Work out the finished part from the listing and answer in its coordinate system (mm). A direction names the side the tool comes from. Round coordinates to 2 decimals unless told otherwise and drop trailing zeros. Write each loop counter-clockwise with the first axis right and the second up, starting at its lowest first coordinate (ties: lowest second). Pieces come first, ordered by that corner, then holes.
1. Find section B-B (x = 37.5). Write down the section's boundary in (y, z).
2. Find section A-A (y = -10). Write down the section's boundary in (x, z), and give its area (3 significant figures).
3. Straight lines are drawn through the part: probe 1 along X at (y, z) = (12, 3.15); probe 2 along Y at (x, z) = (20, 1.75); probe 3 along X at (y, z) = (18, 2.25). For each, find the intervals that lie inside material, in ascending order.
4. A tool of negligible diameter and unlimited length cuts with its end or side. For faces 1 (the face through (-35, 10, 3)), 2 (the face through (-90, -1, 2)), 3 (the face through (-69.5, 17, 3)), from which of +Z, -Z, +X, -X, +Y, -Y can it reach the whole face along a straight path? Write none if from no direction.
5. Find section C-C (x = -20). Write down the section's boundary in (y, z).
6. Flat-ended cylindrical pins translate along their axes: pin 1 Ø1.5 at (x, z) = (-80.5, 1.5) entering from +Y; pin 2 Ø2.5 at (y, z) = (16.5, 2.5) entering from +X. Find the tip coordinate at first contact, or state that the pin passes through.
7. Determine the mould class of faces 4 (the face through (69.5, 17, 3)), 5 (the face through (1.183, -8.145, 2.535)), 6 (the face through (80, 14, 3)), 7 (the face through (72.1, 5.66, 2.54)) for opening direction X: pulls with the +X half, pulls with the -X half, needs draft (parallel to the pull), parting line crosses it, or undercut.
```python
from build123d import *

# Parameters (mm, degrees)
SZKIC1_W                    = 180
SZKIC1_H                    = 40
DODANIE_WYCI_GNI_CIE1_DEPTH = 5
ZAOKR_GLENIE1_R             = 5
SZKIC2_R                    = 2.2
WYTNIJ_WYCI_GNI_CIE1_DEPTH  = 5
SZKIC3_W                    = 20.5
SZKIC3_H                    = 6
WYTNIJ_WYCI_GNI_CIE2_DEPTH  = 10
SZKIC4_R                    = 2.2
WYTNIJ_WYCI_GNI_CIE3_DEPTH  = 10
SZKIC5_W                    = 12
SZKIC5_H                    = 6
WYTNIJ_WYCI_GNI_CIE4_DEPTH  = 93.330926563
ZAOKR_GLENIE2_R             = 2


with BuildPart() as part:
    # Szkic1 → Dodanie-wyciągnięcie1 (new body)
    with BuildSketch(Plane.XY):
        Rectangle(SZKIC1_W, SZKIC1_H)
    extrude(amount=DODANIE_WYCI_GNI_CIE1_DEPTH)

    # Zaokrąglenie1
    zaokr_glenie1_edges = [part.edges().sort_by_distance(p)[0] for p in [
        (90, -20, 2.5),
        (-90, -20, 2.5),
        (-90, 20, 2.5),
        (90, 20, 2.5),
    ]]
    fillet(zaokr_glenie1_edges, radius=ZAOKR_GLENIE1_R)

    # Szkic2 → Wytnij-wyciągnięcie1 (cut)
    with BuildSketch(Plane.XY.offset(5)):
        with Locations((-70, 5)):
            Circle(SZKIC2_R)
        with Locations((-20, 10)):
            Circle(SZKIC2_R)
        with Locations((20, 10)):
            Circle(SZKIC2_R)
        with Locations((70, 5)):
            Circle(SZKIC2_R)
    extrude(amount=-WYTNIJ_WYCI_GNI_CIE1_DEPTH, mode=Mode.SUBTRACT)

    # Szkic3 → Wytnij-wyciągnięcie2 (cut)
    with BuildSketch(Plane.XY.offset(5)):
        with Locations((-79.75, 17)):
            Rectangle(SZKIC3_W, SZKIC3_H)
        with Locations((79.75, 17)):
            Rectangle(SZKIC3_W, SZKIC3_H)
    extrude(amount=-WYTNIJ_WYCI_GNI_CIE2_DEPTH, mode=Mode.SUBTRACT)

    # Szkic4 → Wytnij-wyciągnięcie3 (cut)
    with BuildSketch(Plane.XY.offset(5)):
        with Locations((0, -10)):
            Circle(SZKIC4_R)
    extrude(amount=-WYTNIJ_WYCI_GNI_CIE3_DEPTH, mode=Mode.SUBTRACT)

    # Szkic5 → Wytnij-wyciągnięcie4 (cut, through all)
    with BuildSketch(Plane.XY.offset(5)):
        with Locations((-35, 7)):
            Rectangle(SZKIC5_W, SZKIC5_H)
        with Locations((35, 7)):
            Rectangle(SZKIC5_W, SZKIC5_H)
    extrude(amount=-WYTNIJ_WYCI_GNI_CIE4_DEPTH, mode=Mode.SUBTRACT)

    # Zaokrąglenie2
    zaokr_glenie2_edges = [part.edges().sort_by_distance(p)[0] for p in [
        (-35, 4, 5),
        (35, 4, 5),
    ]]
    fillet(zaokr_glenie2_edges, radius=ZAOKR_GLENIE2_R)


solid = part.part
```
Worked answers:
1. outline: (-20, 0) - (4, 0) - (4, 3) arc R2 ccw to (2, 5) - (-20, 5) - close; (10, 0) - (20, 0) - (20, 5) - (10, 5) - close
2. outline: (-90, 0) - (-2.2, 0) - (-2.2, 5) - (-90, 5) - close; (2.2, 0) - (90, 0) - (90, 5) - (2.2, 5) - close
2. area: 878 mm2
3. probe 1: x = -90 to -20.92, -19.08 to 19.08, 20.92 to 90
3. probe 2: y = -20 to 7.8, 12.2 to 20
3. probe 3: x = -69.5 to 69.5
4. face 1: +Z, -Z
4. face 2: +Z, -Z, -X, +Y, -Y
4. face 3: +Z, -Z, -X, +Y
5. outline: (-20, 0) - (7.8, 0) - (7.8, 5) - (-20, 5) - close; (12.2, 0) - (20, 0) - (20, 5) - (12.2, 5) - close
6. pin 1: stops at y = 14
6. pin 2: stops at x = 69.5
7. face 4: pulls with the +X half
7. face 5: undercut
7. face 6: needs draft
7. face 7: undercut
